Geometry check sheet. Reference: the model listing, model coordinates, mm. A direction names the side the tool comes from. Round coordinates to 2 decimals unless told otherwise and drop trailing zeros. Order: outer loops, then holes, each group sorted by start corner. A loop starts at its lowest first (then second) coordinate and runs counter-clockwise, first axis right, second up.
(1) Cross-section at A-A on z = 12. Enter the section's corners in (x, y).
(2) Cross-section at C-C on y = 39. Enter the section's corners in (x, z), and give its area (3 significant figures).
(3) Cross-section at D-D on x = 45. Enter the section's corners in (y, z).
(4) Set-up check for faces 1 (the face through (-35.594, 6.191, 32.045)), 2 (the face through (-48, 22.5, 32)), 3 (the face through (40, 20, 32)), 4 (the face through (1, -48, -37)), 5 (the face through (-55, 0, 32)): record each of +Z, -Z, +X, -X, +Y, -Y from which the full face is reachable in a straight line by a thin tool's end or side.
(5) Thickness scan on L1, parallel to Z at x = -44, y = -6.5; L2, parallel to X at y = 36, z = -7.5; L3, parallel to Y at x = 20.5, z = 47.5. Record the ranges inside material, lowest first.
(6) Gauge pin test, flat ends, axial feed: P1, Ø1.5, axis at y = -30, z = 11, coming from the +X side; P2, Ø4, axis at x = -13.5, y = 19, coming from the +Z side; P3, Ø6.5, axis at x = 45.5, z = 27.5, coming from the +Y side. Record the tip position at first contact, or that the pin passes through.
(7) Cross-section at B-B on x = 32. Enter the section's corners in (y, z), and give its area (3 significant figures).
(8) Draft check along X on faces 6 (the face through (-59.37, 6.08, 32.04)), 7 (the face through (54, 10, 0)), 8 (the face through (-35.63, 13.92, 32.04)), 9 (the face through (1, -2, 57)). Enter one of: pulls with the +X half, pulls with the -X half, needs draft (parallel to the pull), parting line crosses it, or undercut.
from build123d import *

# Parameters (mm, degrees)
BOSS_EXTRUDE1_DEPTH = 50
BOSS_EXTRUDE3_DEPTH = 65


with BuildPart() as part:
    # Sketch1 → Boss-Extrude1 (new body, symmetric)
    with BuildSketch(Plane(origin=(0, 0, 0), x_dir=(0, 0, -1), z_dir=(1, 0, 0))):
        Polygon((0, 0), (-55, 0), (-60, -5), (-60, -45), (-55, -50), (35, -50), (40, -45), (40, 45), (35, 50), (5, 50), (0, 45), align=None)
    extrude(amount=BOSS_EXTRUDE1_DEPTH, both=True)

    # Sketch2 → Boss-Extrude3 (add)
    with BuildSketch(Plane.XY):
        Polygon((60.643277803, 10), (58.133135104, 17.725424859), (51.561496203, 22.5), (43.438503797, 22.5), (36.866864896, 17.725424859), (34.356722197, 10), (36.866864896, 2.274575141), (43.438503797, -2.5), (51.561496203, -2.5), (58.133135104, 2.274575141), align=None)
    boss_extrude3 = extrude(amount=BOSS_EXTRUDE3_DEPTH)

    # Mirror1: Boss-Extrude3 across plane
    add(boss_extrude3.mirror(Plane(origin=(0, 0, 0), x_dir=(0, 0, 1), z_dir=(1, 0, 0))))


solid = part.part
Found:
1. outline: (-60.64, 10) - (-58.13, 2.27) - (-51.56, -2.5) - (-50, -2.5) - (-50, -50) - (50, -50) - (50, -2.5) - (51.56, -2.5) - (58.13, 2.27) - (60.64, 10) - (58.13, 17.73) - (51.56, 22.5) - (43.44, 22.5) - (36.87, 17.73) - (34.36, 10) - (36.87, 2.27) - (40, 0) - (-40, 0) - (-36.87, 2.27) - (-34.36, 10) - (-36.87, 17.73) - (-43.44, 22.5) - (-51.56, 22.5) - (-58.13, 17.73) - close
2. outline: (-50, -40) - (50, -40) - (50, 0) - (-50, 0) - close
2. area: 4,000 mm2
3. outline: (-50, -35) - (-45, -40) - (45, -40) - (50, -35) - (50, -5) - (45, 0) - (22.5, 0) - (22.5, 65) - (-2.5, 65) - (-2.5, 57.5) - (-5, 60) - (-45, 60) - (-50, 55) - close
4. face 1: +Z
4. face 2: +Z, +X, -X, +Y
4. face 3: +Z, +Y
4. face 4: -Z, +X, -X, -Y
4. face 5: +Z, -Z, -X, -Y
5. L1: z = -40 to 60
5. L2: x = -50 to 50
5. L3: y = -50 to 0
6. P1: stops at x = 50
6. P2: stops at z = 0
6. P3: stops at y = 22.5
7. outline: (-50, -35) - (-45, -40) - (45, -40) - (50, -35) - (50, -5) - (45, 0) - (0, 0) - (0, 55) - (-5, 60) - (-45, 60) - (-50, 55) - close
7. area: 6,940 mm2
8. face 6: pulls with the -X half
8. face 7: needs draft
8. face 8: undercut
8. face 9: undercut
